from build123d import *

# Parameters (mm, degrees)
SKETCH1_W           = 5
SKETCH1_H           = 2
BOSS_EXTRUDE1_DEPTH = 62
FILLET1_R           = 0.5
FILLET2_R           = 1
FILLET3_R           = 0.5


with BuildPart() as part:
    # Sketch1 → Boss-Extrude1 (new body)
    with BuildSketch(Plane(origin=(0, 0, 0), x_dir=(0, 1, 0), z_dir=(0, 0, 1))):
        with Locations((-2.5, -1)):
            Rectangle(SKETCH1_W, SKETCH1_H)
        Polygon((0, -4.886751346), (0, -2), (-5, -2), align=None)
        Polygon((-5, -16.87062059), (-5, -2), (-5, 0), (-8, 0), (-8, -18.87062059), (-5, -18.87062059), align=None)
        Polygon((0, -13.983869244), (-5, -16.87062059), (0, -16.87062059), align=None)
        with Locations((-2.5, -17.87062059)):
            Rectangle(SKETCH1_W, SKETCH1_H)
    extrude(amount=BOSS_EXTRUDE1_DEPTH)

    # Fillet1
    fillet1_edges = [part.edges().sort_by_distance(p)[0] for p in [
        (4.886751346, 0, 31),
        (2, -5, 31),
        (16.87062059, -5, 31),
        (13.983869244, 0, 31),
    ]]
    fillet(fillet1_edges, radius=FILLET1_R)

    # Fillet2
    fillet2_edges = [part.edges().sort_by_distance(p)[0] for p in [
        (18.87062059, 0, 31),
        (18.87062059, -8, 31),
        (0, -8, 31),
        (0, 0, 31),
    ]]
    fillet(fillet2_edges, radius=FILLET2_R)

    # Fillet3
    fillet3_edges = [part.edges().sort_by_distance(p)[0] for p in [
        (9.435310295, -5, 0),
        (9.435310295, -5, 62),
        (15.427244917, -2.5, 0),
        (15.427244917, -2.5, 62),
        (3.443375673, -2.5, 0),
        (3.443375673, -2.5, 62),
        (4.453738644, -0.25, 0),
        (14.416881946, -0.25, 0),
        (4.453738644, -0.25, 62),
        (14.416881946, -0.25, 62),
        (16.437607888, -4.75, 0),
        (16.437607888, -4.75, 62),
        (2.433012702, -4.75, 0),
        (2.433012702, -4.75, 62),
        (16.360257619, 0, 0),
        (16.360257619, 0, 62),
        (18.87062059, -4, 0),
        (9.435310295, -8, 0),
        (0, -4, 0),
        (2.510362971, 0, 0),
        (0.292893219, -0.292893219, 0),
        (0.292893219, -7.707106781, 0),
        (18.577727371, -7.707106781, 0),
        (18.577727371, -0.292893219, 0),
        (18.87062059, -4, 62),
        (2.510362971, 0, 62),
        (0, -4, 62),
        (9.435310295, -8, 62),
        (0.292893219, -0.292893219, 62),
        (0.292893219, -7.707106781, 62),
        (18.577727371, -7.707106781, 62),
        (18.577727371, -0.292893219, 62),
    ]]
    fillet(fillet3_edges, radius=FILLET3_R)


solid = part.part
Input: part model. Units: mm. Frame: model coordinates. A direction names the side the tool comes from. Round coordinates to 2 decimals unless told otherwise and drop trailing zeros. Loops run counter-clockwise (first coordinate to the right, second up) from the corner with the lowest first, then second, coordinate; pieces in that order, holes last. Notation, with made-up numbers: (66, 80) -> (77, 80) arc R19 ccw to (77, 114) -> close; hole circle Ø1 at (-9, 18). An arc over 180 degrees is marked (long way). Answer as a JSON object with one key per item and string values. Group by question number.
1) Ray query, L1, parallel to X at y = -4.5, z = 39.5; L2, parallel to Y at x = 10.5, z = 43; L3, parallel to X at y = -1.5, z = 16. Return the intervals inside material, ascending.
2) Section query A-A on x = 8.25. Output: boundary loops of the cut face in (y, z), plus the area to 3 significant figures.
3) Reachability of faces 1 (the flat face through (15.413, -2.476, 30.573)), 2 (the cylindrical face through (15.565, -2.453, 61.85)), 3 (the cylindrical face through (15.6, -2.4, 0.1)) from +Z, -Z, +X, -X, +Y, -Y: full face, straight path, thin tool, end or side. Return the list, or none.
4) Draft query along Y for faces 4 (the flat face through (18.871, -4, 31)), 5 (the flat face through (3, 0, 31)), 6 (the flat face through (3.43, -2.52, 30.57)). Return one class per face: +Y half, -Y half, draft (parallel to the pull), parting line (faces both ways), or undercut.
5) Section query B-B on z = 56. Output: boundary loops of the cut face in (x, y).
6) Pin query (flat end, axial travel): pin 1 (4 mm diameter, centred on x = 10, z = 32.5, fed in from +Y). Return the tip coordinate at first contact, or that it passes through.
Reply:
{
 "1": {"L1": "x = 0 to 2.37, 16.5 to 18.87", "L2": "y = -8 to -5", "L3": "x = 0 to 4.02, 14.85 to 18.87"},
 "2": {"outline": "(-8, 0.5) arc R0.5 ccw to (-7.5, 0) -> (-5.5, 0) arc R0.5 ccw to (-5, 0.5) -> (-5, 61.5) arc R0.5 ccw to (-5.5, 62) -> (-7.5, 62) arc R0.5 ccw to (-8, 61.5) -> close", "area": "186 mm2"},
 "3": {"face 1": "+Z, -Z", "face 2": "+Z", "face 3": "-Z"},
 "4": {"face 4": "draft", "face 5": "+Y half", "face 6": "undercut"},
 "5": {"outline": "(0, -7) arc R1 ccw to (1, -8) -> (17.87, -8) arc R1 ccw to (18.87, -7) -> (18.87, -1) arc R1 ccw to (17.87, 0) -> (14.85, 0) arc R0.5 ccw to (14.42, -0.75) -> (16.44, -4.25) arc R0.5 cw to (16, -5) -> (2.87, -5) arc R0.5 cw to (2.43, -4.25) -> (4.45, -0.75) arc R0.5 ccw to (4.02, 0) -> (1, 0) arc R1 ccw to (0, -1) -> close"},
 "6": {"pin 1": "stops at y = -5"}
}
